Geometry check sheet. Reference: the model listing, model coordinates, mm. A direction names the side the tool comes from. Round coordinates to 2 decimals unless told otherwise and drop trailing zeros. Order: outer loops, then holes, each group sorted by start corner. A loop starts at its lowest first (then second) coordinate and runs counter-clockwise, first axis right, second up.
(1) Release check for a two-part mould opening along Y. For faces 1 (the face through (13.5, 8, -35)), 2 (the face through (14, 8, 125)), 3 (the face through (7, 13.5, -35)), 4 (the face through (7, 0, -35)) record: +Y half, -Y half, draft (parallel to the pull), parting line (faces both ways), or undercut.
(2) Sectioned sample at A-A (z = 87). Record the boundary of the cut face in (x, y).
(3) Set-up check for faces 5 (the face through (8, 1.5, -35)), 6 (the face through (0, 8, -35)): record each of +Z, -Z, +X, -X, +Y, -Y from which the full face is reachable in a straight line by a thin tool's end or side.
(4) Material ranges on line 1 along Y through (x, z) = (2.5, -36.5); line 2 along X through (y, z) = (14.6, -160), recorded low to high.
Autodesk Inventor part; units mm, degrees
ref_plane "YZ Plane" through (0, 0, 0) normal (1, 0, 0) x (0, 1, 0)
ref_plane "XZ Plane" through (0, 0, 0) normal (0, 1, 0) x (-1, 0, 0)
ref_plane "XY Plane" through (0, 0, 0) normal (0, 0, 1) x (1, 0, 0)
sketch "スケッチ1" plane through (0, 0, 0) normal (0, 0, 1) x (1, 0, 0)
  line L0 (0, 0) -> (15, 0)
  line L1 (15, 0) -> (15, 15)
  line L2 (15, 15) -> (0, 15)
  line L3 (0, 15) -> (0, 0)
  dimension "d0" = 15
  dimension "d1" = 15
extrude "押し出し1" add sketch "スケッチ1" along normal blind 140
sketch "スケッチ2" plane through (0, 15, 0) normal (0, 1, 0) x (1, 0, 0)
  line L0 (0, 0) -> (0, -140) construction
  line L1 (15, -80) -> (15, -65) construction
  line L2 (15, -65) -> (0, -65) construction
  circle A0 centre (7.5, -72.5) radius 1.6
  line L3 (15, 0) -> (15, -140) construction
  line L4 (15, 0) -> (0, 0) construction
  line L5 (0, 0) -> (0, -15) construction
  line L6 (0, -15) -> (15, -15) construction
  line L7 (15, -15) -> (15, 0) construction
  circle A1 centre (7.5, -7.5) radius 1.6
  dimension "d5" = 15
  dimension "d6" = 15
  dimension "d7" = 3.2
  dimension "d8" = 15
  dimension "d9" = 15
  dimension "d10" = 3.2
hole "穴1" at (7.5, 15, 72.5) at (7.5, 15, 7.5) direction (0, -1, 0) diameter 3.2 end through all
sketch "スケッチ3" plane through (0, 0, 0) normal (0, 0, -1) x (-1, 0, 0)
  line L0 (0, 0) -> (-15, 0)
  line L1 (-15, 0) -> (-15, 15)
  line L2 (-15, 15) -> (0, 15)
  line L3 (0, 15) -> (0, 0)
  dimension "d18" = 15
  dimension "d19" = 15
extrude "押し出し2" add sketch "スケッチ3" along normal blind 200
sketch "スケッチ4" plane through (0, 0, -200) normal (0, 0, -1) x (-1, 0, 0)
  point P0 (0, 0)
sketch "スケッチ5" plane through (0, 0, -200) normal (0, 0, -1) x (-1, 0, 0)
  line L0 (0, 0) -> (-15, 0)
  line L1 (0, 0) -> (-15, 0)
  line L2 (-15, 0) -> (-15, 15)
  line L3 (-15, 15) -> (0, 15)
  line L4 (0, 15) -> (0, 0)
  dimension "d22" = 15
  dimension "d23" = 15
extrude "押し出し3" cut sketch "スケッチ5" against normal blind 15
sketch "スケッチ6" plane through (0, 0, -185) normal (0, 0, -1) x (-1, 0, 0)
  line L0 (0, 15) -> (0, 0)
  line L1 (0, 0) -> (-15, 0)
  line L2 (-15, 0) -> (-15, 15)
  line L3 (-15, 15) -> (0, 15)
  line L4 (0, 15) -> (0, 0)
  dimension "d26" = 15
  dimension "d27" = 15
extrude "押し出し4" add sketch "スケッチ6" along normal blind 15
sketch "スケッチ7" plane through (0, 0, 140) normal (0, 0, 1) x (1, 0, 0)
  line L0 (0, 0) -> (15, 0)
  line L1 (15, 0) -> (15, 15)
  line L2 (15, 15) -> (0, 15)
  line L3 (0, 15) -> (0, 0)
  dimension "d30" = 15
  dimension "d31" = 15
extrude "押し出し5" cut sketch "スケッチ7" against normal blind 15
sketch "スケッチ9" plane through (15, 0, -200) normal (1, 0, 0) x (0, 0, -1)
  circle A0 centre (-315, 7.5) radius 1.6
  line L0 (-325, 15) -> (-325, 0)
  line L1 (-325, 0) -> (0, 0)
  point P0 (-200, 0)
  dimension "d44" = 3.2
  dimension "d45" = 10
  dimension "d46" = 7.5
hole "穴3" at (15, 7.5, 115) direction (-1, 0, 0) diameter 3.2 end through all
sketch "スケッチ10" plane through (15, 0, -200) normal (1, 0, 0) x (0, 0, -1)
  circle A0 centre (-315, 7.5) radius 1.6
  line L0 (-325, 0) -> (0, 0)
  point P0 (-200, 0)
  point P1 (-305, 7.5)
  dimension "d54" = 10
  dimension "d55" = 7.5
hole "穴4" at (15, 7.5, 105) direction (-1, 0, 0) diameter 3.2 end through all
sketch "スケッチ11" plane through (15, 0, -200) normal (1, 0, 0) x (0, 0, -1)
  line L0 (0, 15) -> (0, 0)
  line L1 (0, 15) -> (-325, 15)
  point P0 (-200, 0)
  point P1 (-24, 7.5)
  point P2 (-34, 7.5)
  dimension "d63" = 24
  dimension "d64" = 7.5
  dimension "d65" = 10
  dimension "d66" = 7.5
hole "穴5" at (15, 7.5, -166) at (15, 7.5, -176) direction (-1, 0, 0) diameter 3.2 end through all
sketch "スケッチ12" plane through (0, 15, -200) normal (0, 1, 0) x (1, 0, 0)
  line L0 (0, 0) -> (15, 0)
  point P0 (0, -200)
  point P1 (7.5, -40)
  point P2 (7.5, -50)
  point P3 (7.5, -90)
  point P4 (7.5, -100)
  point P5 (7.5, -110)
  point P6 (7.5, -150)
  point P7 (7.5, -160)
  point P8 (7.5, -170)
  dimension "d74" = 40
  dimension "d75" = 7.5
  dimension "d76" = 10
  dimension "d77" = 90
  dimension "d78" = 10
  dimension "d79" = 10
  dimension "d80" = 150
  dimension "d81" = 10
  dimension "d82" = 10
hole "穴6" at (7.5, 15, -30) at (7.5, 15, -40) at (7.5, 15, -50) at (7.5, 15, -90) at (7.5, 15, -100) at (7.5, 15, -110) at (7.5, 15, -150) at (7.5, 15, -160) direction (0, -1, 0) diameter 3.2 end through all
sketch "スケッチ13" plane through (0, 0, 125) normal (0, 0, 1) x (1, 0, 0)
  line L0 (1.5, 13.5) -> (13.5, 13.5)
  line L1 (13.5, 13.5) -> (13.5, 1.5)
  line L2 (13.5, 1.5) -> (1.5, 1.5)
  line L3 (1.5, 1.5) -> (1.5, 13.5)
  line L4 (0, 0) -> (0, 15)
  line L5 (0, 15) -> (15, 15)
  dimension "d90" = 12
  dimension "d91" = 12
  dimension "d92" = 1.5
  dimension "d93" = 1.5
extrude "押し出し6" cut sketch "スケッチ13" against normal blind 340
properties part number "射出_角柱2" material "アルミニウム 6061"
Answer below:
1. face 1: undercut
1. face 2: draft
1. face 3: undercut
1. face 4: -Y half
2. outline: (0, 0) - (15, 0) - (15, 15) - (0, 15) - close; hole (1.5, 1.5) - (13.5, 1.5) - (13.5, 13.5) - (1.5, 13.5) - close
3. face 5: +Z, -Z
3. face 6: +Z, -Z, -X, +Y, -Y
4. line 1: y = 0 to 1.5, 13.5 to 15
4. line 2: x = 0 to 5.9, 9.1 to 15
